Geometry: see drawing. Coordinates: mm, zero at the bounding-box minimum. A direction names the side the tool comes from. Give positions to 0.01 mm unless a question says otherwise; leave off trailing zeros. Write each loop counter-clockwise with the first axis right and the second up, starting at its lowest first coordinate (ties: lowest second). Pieces come first, ordered by that corner, then holes. Notation, with made-up numbers: M 38.5,83.5 L 71.5,83.5 A17 cw 71.5,87.5 Z; hole C 89.25,-28.5 d1. An arc over 180 degrees is marked long. Use CSV: the item, a comma, the result in double quotes. Start each with the question number.
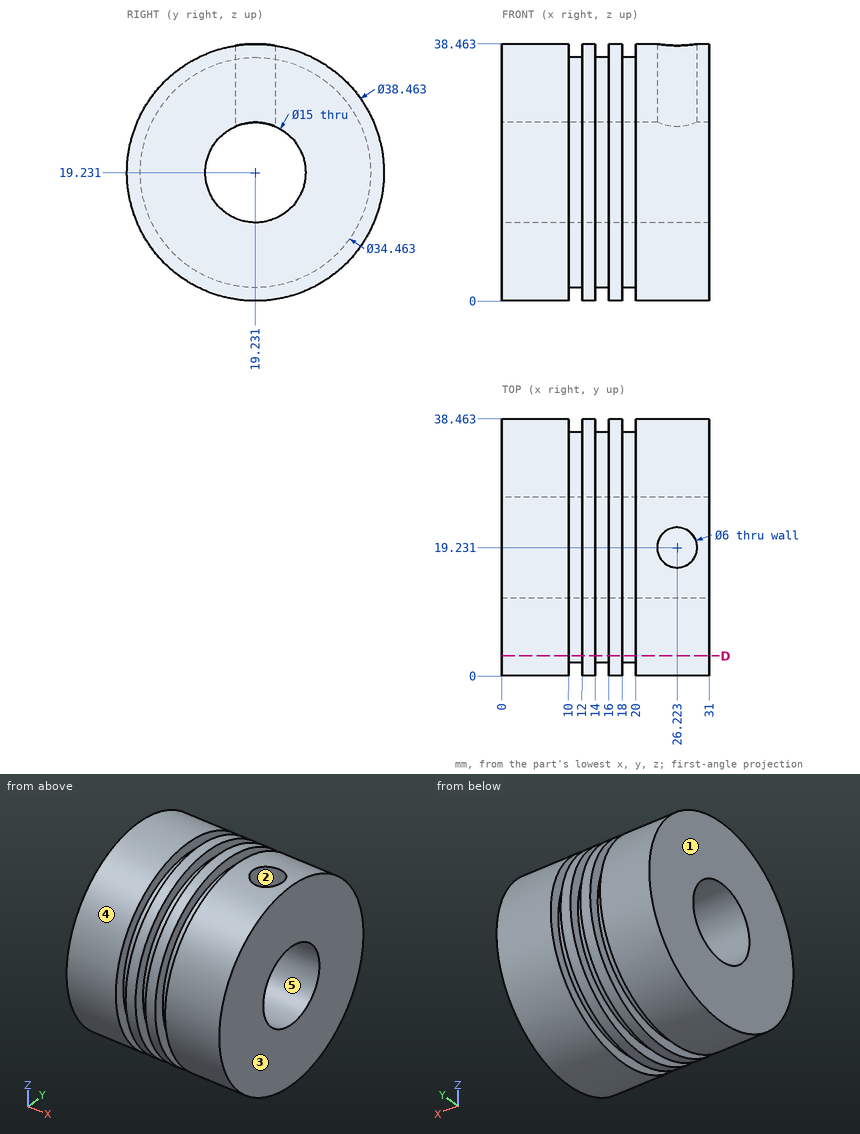
1. First-contact query: pin 1 (10 mm diameter, centred on x = 16, y = 8, fed in from +Z) (1 decimal); pin 2 (1.5 mm diameter, centred on x = 20, z = 9, fed in from +Y); pin 3 (3.5 mm diameter, centred on x = 26.22, y = 19.23, fed in from +Z); pin 4 (12 mm diameter, centred on x = 21, y = 22, fed in from -Z). Flat tips, straight axial feed; report the tip coordinate or a pass-through.
2. Section D-D on y = 3. Return loops of the section in (x, z) (1 decimal), then the cut area to 3 significant figures.
3. Line query: probe 1 along Y at (x, z) = (19.5, 13) (1 decimal); probe 2 along Y at (x, z) = (24, 34.5) (1 decimal); probe 3 along Z at (x, y) = (28, 22.5). Output: solid intervals per line, ascending.
4. Access query for the marked faces 1 and 2. Directions: +Z, -Z, +X, -X, +Y, -Y. A direction counts if a zero-diameter tool reaches every point of the face in a straight line with its end or side. Return the directions, or none.
5. Pull-direction query (Y, two-part tool) for the marked faces 3, 4 and 5; classes: released by +Y, released by -Y, zero draft, split by the parting line, or undercut.
Resolved:
1,pin 1,"stops at z = 37.4"
1,pin 2,"stops at y = 35.96"
1,pin 3,"stops at z = 11.94"
1,pin 4,"stops at z = 0"
2,outline,"M 0,8.9 L 10,8.9 L 10,13.4 L 12,13.4 L 12,8.9 L 14,8.9 L 14,13.4 L 16,13.4 L 16,8.9 L 18,8.9 L 18,13.4 L 20,13.4 L 20,8.9 L 31,8.9 L 31,29.5 L 20,29.5 L 20,25 L 18,25 L 18,29.5 L 16,29.5 L 16,25 L 14,25 L 14,29.5 L 12,29.5 L 12,25 L 10,25 L 10,29.5 L 0,29.5 Z"
2,area,"585 mm2"
3,probe 1,"y = 3.2 to 15.1, 23.4 to 35.3"
3,probe 2,"y = 7.5 to 17.2, 21.2 to 30.9"
3,probe 3,"z = 0.28 to 12.48, 25.98 to 38.18"
4,face 1,"+Z, -Z, -X, +Y, -Y"
4,face 2,"+Z"
5,face 3,"zero draft"
5,face 4,"split by the parting line"
5,face 5,"undercut"
